CAD build for the part. Positions are in the model's coordinates, mm. A direction names the side the tool comes from. Coordinates: 2 decimals unless noted, no trailing zeros. Write each loop counter-clockwise with the first axis right and the second up, starting at its lowest first coordinate (ties: lowest second). Pieces come first, ordered by that corner, then holes. Notation, with made-up numbers: (42, 10) - (68, 10) arc R34 cw to (68, 41) - close; hole circle Ø7 at (37.5, 22.25). An arc over 180 degrees is marked (long way). Answer in a Markdown table with one row per item. Add a question column.
Q1. 3-axis set-ups, long thin cutter, end or side, ignore diameter. For faces 5 (the cylindrical face through (10.42, -8.31, 2.28)), 6 (the cylindrical face through (-10.424, 7.96, 2.097)), 7 (the flat face through (-2, -1, 3.81)), 8 (the flat face through (-3.4, 0.2, 0)): which of +Z, -Z, +X, -X, +Y, -Y reach the whole face in a straight line?
Q2. Drill centre lines: line 1 along Z through (x, y) = (-12.25, -7.62); line 2 along Z through (x, y) = (-12.5, -7.75); line 3 along Y through (x, z) = (9.75, 3.75). Where is each one in solid material? Low to high. Write a range as from..to.
Q3. Two-plate mould, pull along Z, no slides. Class faces 1 (the cylindrical face through (-10.42, -8.62, 2.65)), 2 (the cylindrical face through (-0.44, -1.984, 5.098)), 3 (the conical face through (-6.106, -7.812, 3.132)), 4 (the flat face through (0, 3, 6.35)): +Z half, -Z half, draft (parallel to the pull), parting line (faces both ways), or undercut.
Q4. Band-saw the part on A-A (x = 0). List the corners of the cut face in (y, z), and give its area (3 significant figures).
Q5. Band-saw the part on C-C (z = 5.5). List the corners of the cut face in (x, y).
Q6. Band-saw the part on B-B (y = 0). List the corners of the cut face in (x, z), and give its area (3 significant figures).
Q7. Band-saw the part on D-D (z = 1.5). List the corners of the cut face in (x, y).
Q8. Pin check, flat tips, straight feed: pin 1 (2 mm diameter, centred on y = 7.62, z = 3.175, fed in from -X); pin 2 (1.8 mm diameter, centred on y = -7.62, z = 3.175, fed in from +X); pin 3 (2 mm diameter, centred on x = -1.5, y = 0.5, fed in from -Z). Stop position of each tip, or through.
```python
from build123d import *

# Parameters (mm, degrees)
SKETCH2_W                 = 28.575
SKETCH2_H                 = 25.4
BOSS_EXTRUDE1_DEPTH       = 6.35
F_4_40_TAPPED_HOLE2_D     = 2.2606
F_4_40_TAPPED_HOLE2_DEPTH = 7.62
F_4_40_TAPPED_HOLE2_TIP   = 0.679152758
F_4_40_TAPPED_HOLE1_D     = 2.2606
F_4_40_TAPPED_HOLE1_DEPTH = 7.62
F_4_40_TAPPED_HOLE1_TIP   = 0.679152758
SKETCH7_R                 = 2.032
CUT_EXTRUDE1_DEPTH        = 2.54
SKETCH12_R                = 3.048
CUT_EXTRUDE2_DEPTH        = 3.81


with BuildPart() as part:
    # Sketch2 → Boss-Extrude1 (new body)
    with BuildSketch(Plane.XY):
        Rectangle(SKETCH2_W, SKETCH2_H)
    extrude(amount=BOSS_EXTRUDE1_DEPTH)

    # #4-40 Tapped Hole2
    with Locations(Plane(origin=(14.2875, 0, 0), x_dir=(0, 0, -1), z_dir=(1, 0, 0))):
        with Locations((-3.175, 7.62), (-3.175, -7.62)):
            Hole(F_4_40_TAPPED_HOLE2_D / 2, depth=F_4_40_TAPPED_HOLE2_DEPTH)
            with Locations((0, 0, -(F_4_40_TAPPED_HOLE2_DEPTH + F_4_40_TAPPED_HOLE2_TIP / 2))):  # 118° drill point
                Cone(0, F_4_40_TAPPED_HOLE2_D / 2, F_4_40_TAPPED_HOLE2_TIP, mode=Mode.SUBTRACT)

    # #4-40 Tapped Hole1
    with Locations(Plane.ZY.offset(14.2875)):
        with Locations((3.175, 7.62), (3.175, -7.62)):
            Hole(F_4_40_TAPPED_HOLE1_D / 2, depth=F_4_40_TAPPED_HOLE1_DEPTH)
            with Locations((0, 0, -(F_4_40_TAPPED_HOLE1_DEPTH + F_4_40_TAPPED_HOLE1_TIP / 2))):  # 118° drill point
                Cone(0, F_4_40_TAPPED_HOLE1_D / 2, F_4_40_TAPPED_HOLE1_TIP, mode=Mode.SUBTRACT)

    # Sketch7 → Cut-Extrude1 (cut)
    with BuildSketch(Plane.XY.offset(6.35)):
        Circle(SKETCH7_R)
    extrude(amount=-CUT_EXTRUDE1_DEPTH, mode=Mode.SUBTRACT)

    # Sketch12 → Cut-Extrude2 (cut)
    with BuildSketch(Plane(origin=(0, 0, 0), x_dir=(-1, 0, 0), z_dir=(0, 0, -1))):
        Circle(SKETCH12_R)
    extrude(amount=-CUT_EXTRUDE2_DEPTH, mode=Mode.SUBTRACT)


solid = part.part
```
Checked values:
| question | item | result |
|---|---|---|
| 1 | face 5 | +X |
| 1 | face 6 | -X |
| 1 | face 7 | -Z |
| 1 | face 8 | -Z, +X, -X, +Y, -Y |
| 2 | line 1 | z = 0..2.04, 4.31..6.35 |
| 2 | line 2 | z = 0..2.05, 4.3..6.35 |
| 2 | line 3 | y = -12.7..-8.59, -6.65..6.65, 8.59..12.7 |
| 3 | face 1 | undercut |
| 3 | face 2 | draft |
| 3 | face 3 | undercut |
| 3 | face 4 | +Z half |
| 4 | outline | (-12.7, 0) - (-3.05, 0) - (-3.05, 3.81) - (-2.03, 3.81) - (-2.03, 6.35) - (-12.7, 6.35) - close; (2.03, 3.81) - (3.05, 3.81) - (3.05, 0) - (12.7, 0) - (12.7, 6.35) - (2.03, 6.35) - close |
| 4 | area | 128 mm² |
| 5 | outline | (-14.29, -12.7) - (14.29, -12.7) - (14.29, 12.7) - (-14.29, 12.7) - close; hole circle Ø4.06 at (0, 0) |
| 6 | outline | (-14.29, 0) - (-3.05, 0) - (-3.05, 3.81) - (-2.03, 3.81) - (-2.03, 6.35) - (-14.29, 6.35) - close; (2.03, 3.81) - (3.05, 3.81) - (3.05, 0) - (14.29, 0) - (14.29, 6.35) - (2.03, 6.35) - close |
| 6 | area | 148 mm² |
| 7 | outline | (-14.29, -12.7) - (14.29, -12.7) - (14.29, 12.7) - (-14.29, 12.7) - close; hole circle Ø6.1 at (0, 0) |
| 8 | pin 1 | stops at x = -6.59 |
| 8 | pin 2 | stops at x = 6.53 |
| 8 | pin 3 | stops at z = 3.81 |
